CAD build for the part. Positions are in the model's coordinates, mm. Face numbers are marked on the shaded views. A direction names the side the tool comes from. Give positions to 0.01 mm unless a question says otherwise; leave off trailing zeros. Loops run counter-clockwise (first coordinate to the right, second up) from the corner with the lowest first, then second, coordinate; pieces in that order, holes last. Notation, with made-up numbers: (66, -14.5) - (105, -14.5) arc R23 cw to (105, 22.5) - close; hole circle Ø7 at (23, 51). An arc over 180 degrees is marked (long way). Return JSON: item names as keys, results as strings.
from build123d import *

# Parameters (mm, degrees)
BOSS_EXTRUDE1_DEPTH = 2.97
FILLET1_R           = 0.5
SKETCH2_W           = 10.9
SKETCH2_H           = 1
CUT_EXTRUDE1_DEPTH  = 1.5
CHAMFER1_SIZE       = 2
FILLET2_R           = 1


with BuildPart() as part:
    # Sketch1 → Boss-Extrude1 (new body)
    with BuildSketch(Plane(origin=(0, 0, 0), x_dir=(1, 0, 0), z_dir=(0, 1, 0))):
        with BuildLine():
            Line((5, 0), (5.45, 0))
            Line((5.45, 0), (5.45, 19.6))
            Line((5.45, 19.6), (-5.45, 19.6))
            Line((-5.45, 19.6), (-5.45, 0))
            Line((-5.45, 0), (-5, 0))
            ThreePointArc((-5, 0), (0, 5), (5, 0))
        make_face()
    extrude(amount=BOSS_EXTRUDE1_DEPTH)

    # Fillet1
    # the kernel refuses this fillet: 0.5 mm, written as the material it takes off along each edge
    with BuildSketch(Plane(origin=(5, -1.193063938, 0), x_dir=(1, 0, 0), z_dir=(0, 1, 0))) as fillet1_piece_1:
        with BuildLine():
            CenterArc((0.477225575, 0.5), FILLET1_R, 185.21590857, 84.78409143)
            ThreePointArc((-0.020704023, 0.454545455), (-0.005178688, 0.227508366), (0, 0))
            Line((0, 0), (0.477225575, 0))
        make_face()
    extrude(amount=5.356127875, mode=Mode.SUBTRACT)
    with BuildSketch(Plane(origin=(-5, -1.193063938, 0), x_dir=(-1, 0, 0), z_dir=(0, 1, 0))) as fillet1_piece_2:
        with BuildLine():
            CenterArc((0.477225575, -0.5), FILLET1_R, 90, 84.78409143)
            ThreePointArc((-0.020704023, -0.454545455), (-0.005178688, -0.227508366), (0, 0))
            Line((0, 0), (0.477225575, 0))
        make_face()
    extrude(amount=5.356127875, mode=Mode.SUBTRACT)

    # Sketch2 → Cut-Extrude1 (cut)
    with BuildSketch(Plane(origin=(0, 2.97, 0), x_dir=(1, 0, 0), z_dir=(0, 1, 0))):
        with Locations((0, 18.1)):
            Rectangle(SKETCH2_W, SKETCH2_H)
    extrude(amount=-CUT_EXTRUDE1_DEPTH, mode=Mode.SUBTRACT)

    # Chamfer1
    # the kernel refuses this chamfer: 2 mm, written as the material it takes off along each edge
    with BuildSketch(Plane(origin=(10.593365976, 2.97, -17.6), x_dir=(0, 0.02749587661058627, 0.9996219169112968), z_dir=(-1, 0, 0))) as chamfer1_piece_1_section:
        Polygon((CHAMFER1_SIZE * 0.999621916911, -CHAMFER1_SIZE * 0.0274958766106), (-CHAMFER1_SIZE * 0.0274958766106, -CHAMFER1_SIZE * 0.999621916911), (0, 0), align=None)
    chamfer1_piece_1 = extrude(amount=21.186731952, mode=Mode.PRIVATE)
    chamfer1_piece_1 = split(chamfer1_piece_1, bisect_by=Plane(origin=(0, 1.47, -16.89608178), z_dir=(0, 1, 0)), keep=Keep.TOP, mode=Mode.PRIVATE)
    add(chamfer1_piece_1, mode=Mode.SUBTRACT)

    # Fillet2
    fillet2_edges = [part.edges().sort_by_distance(p)[0] for p in [
        (0, 1.47, -18.6),
        (0, 2.97, -15.6),
    ]]
    fillet(fillet2_edges, radius=FILLET2_R)


solid = part.part
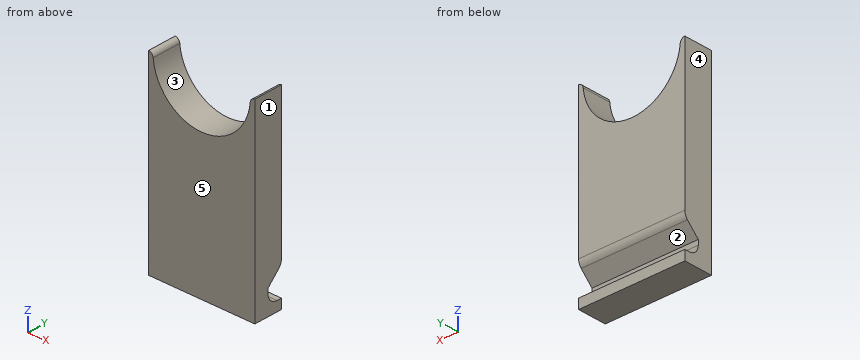
1. Which spindle directions (+Z, -Z, +X, -X, +Y, -Y) get a long thin tool onto all of the face, cutting with end or side? Do the marked faces 1 and 2. Say none if no direction does.
Values follow:
{"face 1": "+Z, -Z, +X, +Y, -Y", "face 2": "+X, -X, +Y"}
2. Pull direction X, two halves, no side cores. Call the marked faces 3, 4 and 5: +X half, -X half, draft (parallel to the pull), parting line (faces both ways), or undercut.
Values follow:
{"face 3": "undercut", "face 4": "-X half", "face 5": "draft"}
3. Cut at B-B, the plane x = 4. Write the cut outline in (y, z).
Values follow:
{"outline": "(0, -19.6) - (2.97, -19.6) - (2.97, -18.6) - (2.47, -18.6) arc R1 cw to (1.47, -17.6) - (1.47, -17.1) - (2.68, -15.89) arc R1 ccw to (2.97, -15.19) - (2.97, -3) - (0, -3) - close"}
4. Cut at A-A, the plane z = -4.75. Write the cut outline in (x, y).
Values follow:
{"outline": "(-5.45, 0) - (-1.56, 0) - (-1.56, 2.97) - (-5.45, 2.97) - close; (1.56, 0) - (5.45, 0) - (5.45, 2.97) - (1.56, 2.97) - close"}
5. Cut at C-C, the plane y = 0.35. Write the cut outline in (x, z), plus the area to 3 significant figures.
Values follow:
{"outline": "(-5.45, -19.6) - (5.45, -19.6) - (5.45, 0) arc R0.5 ccw to (4.98, -0.45) arc R5 cw to (-4.98, -0.45) arc R0.5 ccw to (-5.45, 0) - close", "area": "174 mm²"}
6. Drill centre lines: probe 1 along Z at (x, y) = (-1.75, 2.25); probe 2 along Z at (x, y) = (3, 2.25); probe 3 along X at (y, z) = (0.8, -3). Where is each one in solid material? Low to high.
Values follow:
{"probe 1": "z = -19.6 to -18.58, -16.32 to -4.68", "probe 2": "z = -19.6 to -18.58, -16.32 to -4", "probe 3": "x = -5.45 to -4, 4 to 5.45"}
7. Cut at D-D, the plane x = -0.75. Write the cut outline in (y, z).
Values follow:
{"outline": "(0, -19.6) - (2.97, -19.6) - (2.97, -18.6) - (2.47, -18.6) arc R1 cw to (1.47, -17.6) - (1.47, -17.1) - (2.68, -15.89) arc R1 ccw to (2.97, -15.19) - (2.97, -4.94) - (0, -4.94) - close"}
8. Drop a flat-ended pin along its axis: P1, Ø0.5, axis at x = -2, z = -17.5, coming from the +Y side. Give the stop position or say it passes through.
Values follow:
{"P1": "stops at y = 1.48"}
